Input: part model. Units: mm. Frame: model coordinates. Face numbers are marked on the shaded views. Coordinates: 2 decimals unless noted, no trailing zeros. Loops run counter-clockwise (first coordinate to the right, second up) from the corner with the lowest first, then second, coordinate; pieces in that order, holes last. Notation, with made-up numbers: (-39, 56.25) -> (-32, 56.25) arc R7 ccw to (-32, 61.25) -> close; hole circle Ø6 at (29, 46.5). An arc over 180 degrees is marked (long way). Answer as a JSON object with one key per item and string values.
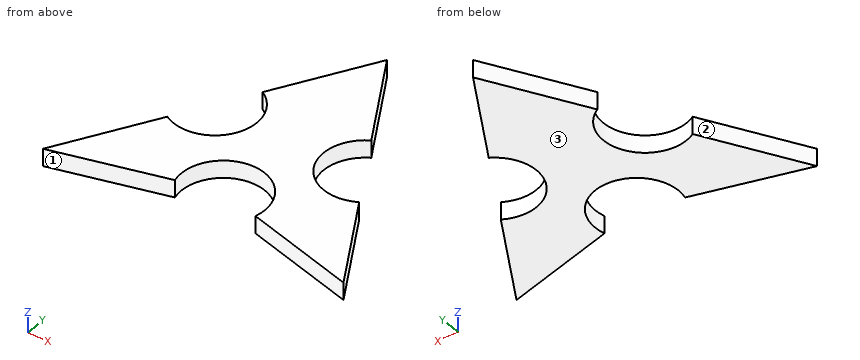
from build123d import *

# Parameters (mm, degrees)
BOSS_EXTRUDE1_DEPTH = 5


with BuildPart() as part:
    # Sketch1 → Boss-Extrude1 (new, symmetric)
    with BuildSketch(Plane.XY):
        with BuildLine():
            Line((31.25, 20.784609691), (0, 74.911197427))
            Line((0, 74.911197427), (0, -27.733592282))
            ThreePointArc((0, -27.733592282), (19.040480167, -37.123317986), (23.182219831, -57.945249365))
            Line((23.182219831, -57.945249365), (86.5, -74.911197427))
            Line((86.5, -74.911197427), (55.25, -20.784609691))
            ThreePointArc((55.25, -20.784609691), (22.465390309, -12), (31.25, 20.784609691))
        make_face()
        with BuildLine():
            Line((0, -27.733592282), (0, 74.911197427))
            Line((0, 74.911197427), (-31.25, 20.784609691))
            ThreePointArc((-31.25, 20.784609691), (-22.465390309, -12), (-55.25, -20.784609691))
            Line((-55.25, -20.784609691), (-86.5, -74.911197427))
            Line((-86.5, -74.911197427), (-23.182219831, -57.945249365))
            ThreePointArc((-23.182219831, -57.945249365), (-19.040480167, -37.123317986), (0, -27.733592282))
        make_face()
    extrude(amount=BOSS_EXTRUDE1_DEPTH, both=True)


solid = part.part
1. Pin query (flat end, axial travel): P1, Ø1, axis at x = -47, z = 3.5, coming from the +Y side; P2, Ø3, axis at y = 7, z = 3, coming from the -X side; P3, Ø6, axis at x = -68, z = 3.5, coming from the -Y side. Return the tip coordinate at first contact, or that it passes through.
Reply:
{"P1": "stops at y = -23.62", "P2": "stops at x = -20.81", "P3": "stops at y = -70.76"}
2. Line query: line 1 along Y through (x, z) = (0, 0); line 2 along X through (y, z) = (-52, -3.5); line 3 along X through (y, z) = (-39.5, -3.5). Output: solid intervals per line, ascending.
Reply:
{"line 1": "y = -27.73 to 74.91", "line 2": "x = -73.27 to -24, 24 to 73.27", "line 3": "x = -66.06 to -20.65, 20.65 to 66.06"}
3. Section query C-C (y = -54). Return loops of the section in (x, z).
Reply:
{"outline": "(-74.43, -5) -> (-23.89, -5) -> (-23.89, 5) -> (-74.43, 5) -> close; (23.89, -5) -> (74.43, -5) -> (74.43, 5) -> (23.89, 5) -> close"}
4. Section query A-A (x = 27.5). Return loops of the section in (y, z), plus the area to 3 significant figures.
Reply:
{"outline": "(-59.1, -5) -> (-18.11, -5) -> (-18.11, 5) -> (-59.1, 5) -> close; (18.11, -5) -> (27.28, -5) -> (27.28, 5) -> (18.11, 5) -> close", "area": "502 mm2"}
5. Mould query, pull axis X, two halves, no side actions, for the marked faces 1, 2 and 3. Classes: pulls with the +X half, pulls with the -X half, needs draft (parallel to the pull), parting line crosses it, or undercut.
Reply:
{"face 1": "undercut", "face 2": "pulls with the -X half", "face 3": "needs draft"}
6. Section query D-D (x = -2.5). Return loops of the section in (y, z).
Reply:
{"outline": "(-27.86, -5) -> (70.58, -5) -> (70.58, 5) -> (-27.86, 5) -> close"}
